from build123d import *

# Parameters (mm, degrees)
BOSS_EXTRUDE1_DEPTH     = 97
SKETCH2_R               = 2.05
CUT_EXTRUDE1_DEPTH      = 98
SKETCH5_W               = 41.197318768
SKETCH5_H               = 41
CUT_EXTRUDE2_DEPTH      = 60.079477801
CUT_EXTRUDE2_DEPTH_BACK = 29.495236192
CUT_EXTRUDE4_START      = -4
SKETCH6_R               = 2.05
CUT_EXTRUDE4_DEPTH      = 20


with BuildPart() as part:
    # Sketch1 → Boss-Extrude1 (new body)
    with BuildSketch(Plane(origin=(0, 0, 0), x_dir=(1, 0, 0), z_dir=(0, 1, 0))):
        with BuildLine():
            Line((-1.956295201, 0.415823382), (-41.082199231, 8.732291014))
            Line((-41.082199231, 8.732291014), (-58, 0))
            Line((-58, 0), (-59.184498234, -0.611390536))
            ThreePointArc((-59.184498234, -0.611390536), (-59.697587059, -1.73599845), (-58.725833628, -2.5))
            Line((-58.725833628, -2.5), (7.92143542, -2.5))
            Line((7.92143542, -2.5), (8.377039367, -2.5))
            ThreePointArc((8.377039367, -2.5), (15.448107179, 0.428932188), (18.377039367, 7.5))
            Line((18.377039367, 7.5), (18.377039367, 47.131925559))
            ThreePointArc((18.377039367, 47.131925559), (14.674810753, 51.243366322), (10.199141157, 47.990855979))
            Line((10.199141157, 47.990855979), (7.92143542, 37.267423588))
            Line((7.92143542, 37.267423588), (0.415823382, 1.956295201))
            ThreePointArc((0.415823382, 1.956295201), (-0.45119375, 0.694777447), (-1.956295201, 0.415823382))
        make_face()
    extrude(amount=BOSS_EXTRUDE1_DEPTH)

    # Sketch2 → Cut-Extrude1 (cut, through all)
    with BuildSketch(Plane(origin=(0, 97, 0), x_dir=(1, 0, 0), z_dir=(0, 1, 0))):
        with Locations((-45.407004093, 2)):
            Circle(SKETCH2_R)
        with Locations((9.444671894, 5.955813006)):
            Circle(SKETCH2_R)
        with Locations((14.242983228, 47.131925559)):
            Circle(SKETCH2_R)
        with Locations((-30.580095712, 2)):
            Circle(SKETCH2_R)
    extrude(amount=-CUT_EXTRUDE1_DEPTH, mode=Mode.SUBTRACT)

    # Sketch5 → Cut-Extrude2 (cut, two sides)
    with BuildSketch(Plane(origin=(-9.781476007, 0, -2.079116908), x_dir=(-0.207911691, 0, 0.978147601), z_dir=(-0.978147601, 0, -0.207911691))) as cut_extrude2_sk:
        with Locations((-32.598659384, 48.5)):
            Rectangle(SKETCH5_W, SKETCH5_H)
    extrude(amount=CUT_EXTRUDE2_DEPTH, mode=Mode.SUBTRACT)
    extrude(cut_extrude2_sk.sketch, amount=-CUT_EXTRUDE2_DEPTH_BACK, mode=Mode.SUBTRACT)

    # Sketch6 → Cut-Extrude4 (cut)
    with BuildSketch(Plane.XZ.offset(CUT_EXTRUDE4_START)):
        with BuildLine():
            Line((18.377039367, -47.131925559), (18.377039367, -42.783410889))
            ThreePointArc((18.377039367, -42.783410889), (13.61624642, -41.164748591), (9.295652814, -43.737235327))
            Line((9.295652814, -43.737235327), (10.199141157, -47.990855979))
            ThreePointArc((10.199141157, -47.990855979), (14.674810753, -51.243366322), (18.377039367, -47.131925559))
        make_face()
        with Locations((14.242983228, -47.131925559)):
            Circle(SKETCH6_R, mode=Mode.SUBTRACT)
        with BuildLine():
            ThreePointArc((9.295652814, -43.737235327), (12.465904513, -52.862718807), (20.242983228, -47.131925559))
            ThreePointArc((20.242983228, -47.131925559), (19.756799367, -44.765951852), (18.377039367, -42.783410889))
            Line((18.377039367, -42.783410889), (18.377039367, -47.131925559))
            ThreePointArc((18.377039367, -47.131925559), (14.674810753, -51.243366322), (10.199141157, -47.990855979))
            Line((10.199141157, -47.990855979), (9.295652814, -43.737235327))
        make_face()
    extrude(amount=-CUT_EXTRUDE4_DEPTH, mode=Mode.SUBTRACT)


solid = part.part
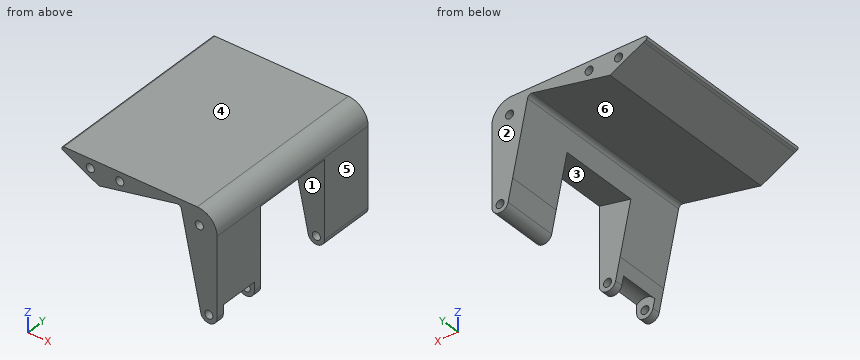
Geometry check sheet. Reference: the model listing, model coordinates, mm. Face numbers are marked on the shaded views. A direction names the side the tool comes from. Coordinates: 2 decimals unless noted, no trailing zeros. Order: outer loops, then holes, each group sorted by start corner. A loop starts at its lowest first (then second) coordinate and runs counter-clockwise, first axis right, second up. Notation, with made-up numbers: M 76.25,24.25 L 82.25,24.25 A32 cw 82.25,63.25 Z; hole C -11.75,31.5 d5. An arc over 180 degrees is marked long. Use CSV: the item, a comma, the result in double quotes.
Item 1: Cross-section at C-C on y = 17. Record the cut outline in (x, z).
Returned:
outline,"M -59.18,0.61 L -41.08,-8.73 L -1.96,-0.42 A2 cw 0.42,-1.96 L 7.92,-37.27 L 9.3,-43.74 A6 cw 18.38,-42.78 L 18.38,-7.5 A10 ccw 8.38,2.5 L -58.73,2.5 A1 ccw Z; hole C -45.41,-2 d4.1; hole C -30.58,-2 d4.1; hole C 9.44,-5.96 d4.1"
Item 2: Cross-section at A-A on y = 82. Record the cut outline in (x, z), then the cut area to 3 significant figures.
Returned:
outline,"M -59.18,0.61 L -41.08,-8.73 L -1.96,-0.42 A2 cw 0.42,-1.96 L 7.92,-37.27 L 10.2,-47.99 A4.13 ccw 18.38,-47.13 L 18.38,-7.5 A10 ccw 8.38,2.5 L -58.73,2.5 A1 ccw Z; hole C -45.41,-2 d4.1; hole C -30.58,-2 d4.1; hole C 9.44,-5.96 d4.1; hole C 14.24,-47.13 d4.1"
area,"1,030 mm2"
Item 3: Thickness scan on line 1 along Y through (x, z) = (8.5, -19.5); line 2 along Z through (x, y) = (-46, 74); line 3 along Z through (x, y) = (13, 80.5). Record the ranges inside material, lowest first.
Returned:
line 1,"y = 0 to 28, 69 to 97"
line 2,"z = -6.19 to -3.96, -0.04 to 2.5"
line 3,"z = -51.07 to -48.76, -45.5 to 1.37"
Item 4: Gauge pin test, flat ends, axial feed: pin 1 Ø5 at (y, z) = (41, -15) entering from -X; pin 2 Ø1.5 at (x, y) = (-44, 82) entering from -Z; pin 3 Ø12 at (x, y) = (-16, 16) entering from -Z; pin 4 Ø10 at (y, z) = (47, -14.5) entering from -X. Record the tip position at first contact, or that the pin passes through.
Returned:
pin 1,"passes through"
pin 2,"stops at z = -7.61"
pin 3,"stops at z = -4.68"
pin 4,"stops at x = 2.02"
Item 5: Mould release check, pull along Y, two halves, no side actions. Record for the marked faces 1, 2, 3 and 4: pulls with the +Y half, pulls with the -Y half, needs draft (parallel to the pull), parting line crosses it, or undercut.
Returned:
face 1,"undercut"
face 2,"pulls with the +Y half"
face 3,"undercut"
face 4,"needs draft"
Item 6: Cross-section at B-B on z = -32.5. Record the cut outline in (x, y).
Returned:
outline,"M 6.91,0 L 18.38,0 L 18.38,28 L 6.91,28 Z; M 6.91,69 L 18.38,69 L 18.38,97 L 6.91,97 Z"
Item 7: Cross-section at D-D on x = 6. Record the cut outline in (y, z), then the cut area to 3 significant figures.
Returned:
outline,"M 0,-28.23 L 28,-28.23 L 28,-10.99 L 69,-10.99 L 69,-28.23 L 97,-28.23 L 97,2.5 L 0,2.5 Z"
area,"2,270 mm2"
Item 8: Tool access check on the marked faces 5 and 6. Record the directions out of +Z, -Z, +X, -X, +Y, -Y that give a thin tool (end or side, any length) a straight path to the whole face; none if there is none.
Returned:
face 5,"+Z, -Z, +X, +Y, -Y"
face 6,"-Z, +Y, -Y"
